from build123d import *

# Parameters (mm, degrees)
SKIZZE1_W                                           = 100
SKIZZE1_H                                           = 100
AUFSATZ_LINEAR_AUSTRAGEN1_DEPTH                     = 200
STIRNSENKUNG_F_R_M8_SENKSCHRAUBE_KOPF_B_D           = 9
STIRNSENKUNG_F_R_M8_SENKSCHRAUBE_KOPF_B_CBORE_D     = 22
STIRNSENKUNG_F_R_M8_SENKSCHRAUBE_KOPF_B_CBORE_DEPTH = 8
KERNLOCH_F_R_M8X1_252_D                             = 6.8
KERNLOCH_F_R_M8X1_252_DEPTH                         = 30
KERNLOCH_F_R_M8X1_252_TIP                           = 2.042926105
KERNLOCH_F_R_M81_D                                  = 6.8
KERNLOCH_F_R_M81_DEPTH                              = 30
KERNLOCH_F_R_M81_TIP                                = 2.042926105
STIRNSENKUNG_F_R_M8_SENKSCHRAUBE_KO_2_D             = 9
STIRNSENKUNG_F_R_M8_SENKSCHRAUBE_KO_2_CBORE_D       = 15
STIRNSENKUNG_F_R_M8_SENKSCHRAUBE_KO_2_CBORE_DEPTH   = 8


with BuildPart() as part:
    # Skizze1 → Aufsatz-Linear austragen1 (new body)
    with BuildSketch(Plane.XY):
        Rectangle(SKIZZE1_W, SKIZZE1_H)
    extrude(amount=AUFSATZ_LINEAR_AUSTRAGEN1_DEPTH)

    # Stirnsenkung f_r M8 Senkschraube _Kopf B (through all)
    with Locations(Plane(origin=(0, 50, 0), x_dir=(1, 0, 0), z_dir=(0, 1, 0))):
        with Locations((0, -175)):
            stirnsenkung_f_r_m8_senkschraube_kopf_b = CounterBoreHole(STIRNSENKUNG_F_R_M8_SENKSCHRAUBE_KOPF_B_D / 2, STIRNSENKUNG_F_R_M8_SENKSCHRAUBE_KOPF_B_CBORE_D / 2, STIRNSENKUNG_F_R_M8_SENKSCHRAUBE_KOPF_B_CBORE_DEPTH)

    # Spiegeln1: Stirnsenkung f_r M8 Senkschraube _Kopf B across plane
    add(stirnsenkung_f_r_m8_senkschraube_kopf_b.mirror(Plane.XY.offset(100)), mode=Mode.SUBTRACT)

    # Kernloch für M8x1.252
    with Locations(Plane(origin=(0, 0, 0), x_dir=(-1, 0, 0), z_dir=(0, 0, -1))):
        with Locations((-30, 0), (30, 0)):
            Hole(KERNLOCH_F_R_M8X1_252_D / 2, depth=KERNLOCH_F_R_M8X1_252_DEPTH)
            with Locations((0, 0, -(KERNLOCH_F_R_M8X1_252_DEPTH + KERNLOCH_F_R_M8X1_252_TIP / 2))):  # 118° drill point
                Cone(0, KERNLOCH_F_R_M8X1_252_D / 2, KERNLOCH_F_R_M8X1_252_TIP, mode=Mode.SUBTRACT)

    # Kernloch für M81
    with Locations(Plane.XY.offset(200)):
        with Locations((30, 0), (-30, 0)):
            Hole(KERNLOCH_F_R_M81_D / 2, depth=KERNLOCH_F_R_M81_DEPTH)
            with Locations((0, 0, -(KERNLOCH_F_R_M81_DEPTH + KERNLOCH_F_R_M81_TIP / 2))):  # 118° drill point
                Cone(0, KERNLOCH_F_R_M81_D / 2, KERNLOCH_F_R_M81_TIP, mode=Mode.SUBTRACT)

    # Stirnsenkung f_r M8 Senkschraube _Ko 2 (through all)
    with Locations(Plane(origin=(0, -50, 0), x_dir=(-1, 0, 0), z_dir=(0, -1, 0))):
        with Locations((0, -175), (0, -25)):
            CounterBoreHole(STIRNSENKUNG_F_R_M8_SENKSCHRAUBE_KO_2_D / 2, STIRNSENKUNG_F_R_M8_SENKSCHRAUBE_KO_2_CBORE_D / 2, STIRNSENKUNG_F_R_M8_SENKSCHRAUBE_KO_2_CBORE_DEPTH)


solid = part.part
Input: part model. Units: mm. Frame: model coordinates. A direction names the side the tool comes from. Coordinates: 2 decimals unless noted, no trailing zeros. Loops run counter-clockwise (first coordinate to the right, second up) from the corner with the lowest first, then second, coordinate; pieces in that order, holes last.
Q1. Cut plane B-B (x = 0). Output: boundary loops of the cut face in (y, z).
Q2. Set-up query: faces 4 (the face through (-1, 1, 0)), 5 (the face through (0.976, -46.056, 167.564)), 6 (the face through (-1.432, 46.056, 164.094)), 7 (the face through (-33.14, -1.3, 184.79)), 8 (the face through (-26.757, 1.021, 15.21)). Return all of +Z, -Z, +X, -X, +Y, -Y with unobstructed straight access to the full face (end or side cutting, diameter ignored); none if empty.
Q3. Material intervals for line 1 (Z direction, x = 0, y = 24); line 2 (X direction, y = 0, z = 185.75); line 3 (Z direction, x = 0, y = 44.25), sorted ascending.
Q4. Cut plane A-A (z = 175). Output: boundary loops of the cut face in (x, y).
Q5. Contact query for flat-ended pins moving along their axis: pin 1 (11 mm diameter, centred on x = -2, z = 170.5, fed in from +Y); pin 2 (14.5 mm diameter, centred on x = 0, z = 25, fed in from -Y); pin 3 (4 mm diameter, centred on x = -30, y = 0, fed in from +Z). Output: stop coordinate, or through.
Q6. Draft query along Z for faces 1 (the face through (0.976, -46.056, 17.564)), 2 (the face through (50, -1, 99)), 3 (the face through (-30.56, 0.18, 31.69)). Return one class per face: +Z half, -Z half, draft (parallel to the pull), parting line (faces both ways), or undercut.
Working result:
1. outline: (-50, 0) - (50, 0) - (50, 14) - (42, 14) - (42, 20.5) - (-42, 20.5) - (-42, 17.5) - (-50, 17.5) - close; (-50, 32.5) - (-42, 32.5) - (-42, 29.5) - (42, 29.5) - (42, 36) - (50, 36) - (50, 164) - (42, 164) - (42, 170.5) - (-42, 170.5) - (-42, 167.5) - (-50, 167.5) - close; (-50, 182.5) - (-42, 182.5) - (-42, 179.5) - (42, 179.5) - (42, 186) - (50, 186) - (50, 200) - (-50, 200) - close
2. face 4: -Z, +X, -X, +Y, -Y
2. face 5: -Y
2. face 6: +Y
2. face 7: +Z
2. face 8: -Z
3. line 1: z = 0 to 20.5, 29.5 to 170.5, 179.5 to 200
3. line 2: x = -50 to -33.4, -26.6 to 26.6, 33.4 to 50
3. line 3: z = 0 to 14, 36 to 164, 186 to 200
4. outline: (-50, -50) - (-7.5, -50) - (-7.5, -42) - (-4.5, -42) - (-4.5, 42) - (-11, 42) - (-11, 50) - (-50, 50) - close; (4.5, -42) - (7.5, -42) - (7.5, -50) - (50, -50) - (50, 50) - (11, 50) - (11, 42) - (4.5, 42) - close; hole circle Ø6.8 at (-30, 0); hole circle Ø6.8 at (30, 0)
5. pin 1: stops at y = 42
5. pin 2: stops at y = -42
5. pin 3: stops at z = 169.16
6. face 1: undercut
6. face 2: draft
6. face 3: -Z half
